```python
from build123d import *

# Parameters (mm, degrees)
SKETCH1_R           = 5.25
SKETCH1_R_2         = 2
SKETCH1_R_3         = 2.5
BOSS_EXTRUDE1_DEPTH = 8


with BuildPart() as part:
    # Sketch1 → Boss-Extrude1 (new body)
    with BuildSketch(Plane(origin=(0, 0, 0), x_dir=(1, 0, 0), z_dir=(0, 1, 0))):
        with BuildLine():
            Line((-167.5, -100), (-150, -117.5))
            Line((-150, -117.5), (150, -117.5))
            Line((150, -117.5), (167.5, -100))
            Line((167.5, -100), (167.5, -97))
            Line((167.5, -97), (150, -97))
            ThreePointArc((150, -97), (143, -90), (150, -83))
            Line((150, -83), (167.5, -83))
            Line((167.5, -83), (167.5, 83))
            Line((167.5, 83), (150, 83))
            ThreePointArc((150, 83), (143, 90), (150, 97))
            Line((150, 97), (167.5, 97))
            Line((167.5, 97), (167.5, 100))
            Line((167.5, 100), (150, 117.5))
            Line((150, 117.5), (-150, 117.5))
            Line((-150, 117.5), (-167.5, 100))
            Line((-167.5, 100), (-167.5, 97))
            Line((-167.5, 97), (-150, 97))
            ThreePointArc((-150, 97), (-143, 90), (-150, 83))
            Line((-150, 83), (-167.5, 83))
            Line((-167.5, 83), (-167.5, -83))
            Line((-167.5, -83), (-150, -83))
            ThreePointArc((-150, -83), (-143, -90), (-150, -97))
            Line((-150, -97), (-167.5, -97))
            Line((-167.5, -97), (-167.5, -100))
        make_face()
        with Locations(Location((-156, 0, 0), (0, 0, 270))):
            Circle(SKETCH1_R, mode=Mode.SUBTRACT)
        with Locations(Location((-156, -10.246017435, 0), (0, 0, 270))):
            Circle(SKETCH1_R_2, mode=Mode.SUBTRACT)
        with Locations(Location((-84.5, 84.5, 0), (0, 0, 270))):
            Circle(SKETCH1_R_3, mode=Mode.SUBTRACT)
        with Locations(Location((0, 84.5, 0), (0, 0, 270))):
            Circle(SKETCH1_R_3, mode=Mode.SUBTRACT)
        with Locations(Location((84.5, 84.5, 0), (0, 0, 270))):
            Circle(SKETCH1_R_3, mode=Mode.SUBTRACT)
        with Locations(Location((84.5, -84.5, 0), (0, 0, 270))):
            Circle(SKETCH1_R_3, mode=Mode.SUBTRACT)
        with Locations(Location((0, -84.5, 0), (0, 0, 270))):
            Circle(SKETCH1_R_3, mode=Mode.SUBTRACT)
        with Locations(Location((-84.5, -84.5, 0), (0, 0, 270))):
            Circle(SKETCH1_R_3, mode=Mode.SUBTRACT)
        with Locations(Location((-156, 10.246017435, 0), (0, 0, 90))):
            Circle(SKETCH1_R_2, mode=Mode.SUBTRACT)
        with Locations(Location((156, 10.246017435, 0), (0, 0, 270))):
            Circle(SKETCH1_R_2, mode=Mode.SUBTRACT)
        with Locations(Location((156, -10.246017435, 0), (0, 0, 90))):
            Circle(SKETCH1_R_2, mode=Mode.SUBTRACT)
        with Locations(Location((156, 0, 0), (0, 0, 90))):
            Circle(SKETCH1_R, mode=Mode.SUBTRACT)
        with Locations(Location((-150, -74, 0), (0, 0, 270))):
            Circle(SKETCH1_R_3, mode=Mode.SUBTRACT)
        with Locations(Location((-134, -90, 0), (0, 0, 270))):
            Circle(SKETCH1_R_3, mode=Mode.SUBTRACT)
        with Locations(Location((-150, -106, 0), (0, 0, 270))):
            Circle(SKETCH1_R_3, mode=Mode.SUBTRACT)
        with Locations(Location((-150, 74, 0), (0, 0, 90))):
            Circle(SKETCH1_R_3, mode=Mode.SUBTRACT)
        with Locations(Location((-134, 90, 0), (0, 0, 90))):
            Circle(SKETCH1_R_3, mode=Mode.SUBTRACT)
        with Locations(Location((-150, 106, 0), (0, 0, 90))):
            Circle(SKETCH1_R_3, mode=Mode.SUBTRACT)
        with Locations(Location((150, -74, 0), (0, 0, 90))):
            Circle(SKETCH1_R_3, mode=Mode.SUBTRACT)
        with Locations(Location((134, -90, 0), (0, 0, 90))):
            Circle(SKETCH1_R_3, mode=Mode.SUBTRACT)
        with Locations(Location((150, -106, 0), (0, 0, 90))):
            Circle(SKETCH1_R_3, mode=Mode.SUBTRACT)
        with Locations(Location((150, 106, 0), (0, 0, 270))):
            Circle(SKETCH1_R_3, mode=Mode.SUBTRACT)
        with Locations(Location((150, 74, 0), (0, 0, 270))):
            Circle(SKETCH1_R_3, mode=Mode.SUBTRACT)
        with Locations(Location((134, 90, 0), (0, 0, 270))):
            Circle(SKETCH1_R_3, mode=Mode.SUBTRACT)
        with BuildLine():
            Line((-80, -60), (80, -60))
            ThreePointArc((80, -60), (87.071067812, -57.071067812), (90, -50))
            Line((90, -50), (90, 50))
            ThreePointArc((90, 50), (87.071067812, 57.071067812), (80, 60))
            Line((80, 60), (-80, 60))
            ThreePointArc((-80, 60), (-87.071067812, 57.071067812), (-90, 50))
            Line((-90, 50), (-90, -50))
            ThreePointArc((-90, -50), (-87.071067812, -57.071067812), (-80, -60))
        make_face(mode=Mode.SUBTRACT)
    extrude(amount=BOSS_EXTRUDE1_DEPTH)


solid = part.part
```
Model file for the job. Use its own axes, mm. A direction names the side the tool comes from. Give positions to 0.01 mm unless a question says otherwise; leave off trailing zeros. Write each loop counter-clockwise with the first axis right and the second up, starting at its lowest first coordinate (ties: lowest second). Pieces come first, ordered by that corner, then holes. Notation, with made-up numbers: (-15, 52) - (16, 52) arc R19 cw to (16, 67) - close; hole circle Ø6 at (6, 58.5). An arc over 180 degrees is marked (long way). One line per question, with ' | ' between items. Start each with the question number.
(1) Slice it at D-D on y = 2.25. Give the number of separate pieces and of enclosed holes in the cut face, plus the area to 3 significant figures.
(2) Slice it at A-A on z = -56. Write the cut outline in (x, y).
(3) Slice it at C-C on x = 56. Write the cut outline in (y, z), plus the area to 3 significant figures.
(4) Slice it at B-B on z = 0. Write the cut outline in (x, y), plus the area to 3 significant figures.
(5) Pin check, flat tips, straight feed: P1, Ø2.5, axis at x = -155, y = 3, coming from the +Z side; P2, Ø2.5, axis at x = -158.5, y = 4.5, coming from the +Z side; P3, Ø12, axis at x = 82, z = -18.5, coming from the -Y side; P4, Ø2.5, axis at x = 160.5, y = 3, coming from the -Z side. Stop position of each tip, or through.
(6) 3-axis set-ups, long thin cutter, end or side, ignore diameter. For faces 5 (the face through (-159, 4, -83)), 6 (the face through (-86.99, 3.94, -57.15)), 7 (the face through (159, 4, 97)), 8 (the face through (-2, 0, 77)): which of +Z, -Z, +X, -X, +Y, -Y reach the whole face in a straight line?
(7) Wall check: line 1 along Z through (x, y) = (-134, 6); line 2 along X through (y, z) = (5.75, 74); line 3 along X through (y, z) = (4, -84.5). Give the ranges that are in metal, low to high. Write a range as from..to.
(8) Two-plate mould, pull along Z, no slides. Class faces 1 (the face through (167.5, 4, 1)), 2 (the face through (-143, 4, -90)), 3 (the face through (158.6, 3.9, 108.9)), 4 (the face through (2, 4, -117.5)): +Z half, -Z half, draft (parallel to the pull), parting line (faces both ways), or undercut.
Results below:
1) separate pieces: 1 | enclosed holes: 25 | area: 54,700 mm^2
2) outline: (-167.5, 0) - (-88, 0) - (-88, 8) - (-167.5, 8) - close; (88, 0) - (167.5, 0) - (167.5, 8) - (88, 8) - close
3) outline: (0, -117.5) - (8, -117.5) - (8, -60) - (0, -60) - close; (0, 60) - (8, 60) - (8, 117.5) - (0, 117.5) - close | area: 920 mm^2
4) outline: (-167.5, 0) - (-161.25, 0) - (-161.25, 8) - (-167.5, 8) - close; (-150.75, 0) - (-90, 0) - (-90, 8) - (-150.75, 8) - close; (90, 0) - (150.75, 0) - (150.75, 8) - (90, 8) - close; (161.25, 0) - (167.5, 0) - (167.5, 8) - (161.25, 8) - close | area: 1,070 mm^2
5) P1: z = 113.75 | P2: z = 110.25 | P3: through | P4: z = -108.25
6) face 5: -X, +Y, -Y | face 6: +Y, -Y | face 7: +X, +Y, -Y | face 8: +Z, -Z, +X, -X, -Y
7) line 1: -117.5..-92.5, -87.5..87.5, 92.5..117.5 | line 2: -167.5..-152.5, -147.5..147.5, 152.5..167.5 | line 3: -145.67..-87, -82..-2.5, 2.5..82, 87..145.67
8) face 1: draft | face 2: undercut | face 3: +Z half | face 4: -Z half
